```python
from build123d import *

# Parameters (mm, degrees)
CROQUIS1_R              = 2.159
CROQUIS1_W              = 21.082
CROQUIS1_H              = 21.082
SALIENTE_EXTRUIR1_DEPTH = 4.445
REDONDEO1_R             = 3.175
REDONDEO2_R             = 1.016
CHAFL_N1_SIZE           = 0.508


with BuildPart() as part:
    # Croquis1 → Saliente-Extruir1 (new body)
    with BuildSketch(Plane(origin=(0, 0, 0), x_dir=(1, 0, 0), z_dir=(0, 1, 0))):
        with BuildLine():
            Line((11.504506555, 42.935402979), (5.259202996, 19.62761279))
            ThreePointArc((5.259202996, 19.62761279), (-14.368409794, -14.368409794), (19.62761279, 5.259202996))
            Line((19.62761279, 5.259202996), (42.935402979, 11.504506555))
            ThreePointArc((42.935402979, 11.504506555), (31.430896424, 31.430896424), (11.504506555, 42.935402979))
        make_face()
        with Locations(Location((22.86, 9.652, 0), (0, 0, 270))):
            Circle(CROQUIS1_R, mode=Mode.SUBTRACT)
        Rectangle(CROQUIS1_W, CROQUIS1_H, mode=Mode.SUBTRACT)
    extrude(amount=SALIENTE_EXTRUIR1_DEPTH)

    # Redondeo1
    redondeo1_edges = [part.edges().sort_by_distance(p)[0] for p in [
        (42.935402979, 2.2225, -11.504506555),
        (19.62761279, 2.2225, -5.259202996),
        (5.259202996, 2.2225, -19.62761279),
        (11.504506555, 2.2225, -42.935402979),
    ]]
    fillet(redondeo1_edges, radius=REDONDEO1_R)

    # Redondeo2
    redondeo2_edges = [part.edges().sort_by_distance(p)[0] for p in [
        (10.541, 2.2225, 10.541),
        (10.541, 2.2225, -10.541),
        (-10.541, 2.2225, -10.541),
        (-10.541, 2.2225, 10.541),
    ]]
    fillet(redondeo2_edges, radius=REDONDEO2_R)

    # Chaflán1
    chafl_n1_edges = [part.edges().sort_by_distance(p)[0] for p in [
        (22.86, 0, -11.811),
        (22.86, 4.445, -11.811),
    ]]
    chamfer(chafl_n1_edges, length=CHAFL_N1_SIZE)


solid = part.part
```
Work out the finished part from the listing and answer in its coordinate system (mm). A direction names the side the tool comes from. Coordinates: 2 decimals unless noted, no trailing zeros. Loops run counter-clockwise (first coordinate to the right, second up) from the corner with the lowest first, then second, coordinate; pieces in that order, holes last.
1) Section D-D (z = -18.5) is taken. Give the vertices of the cut face in (x, y) (1 decimal), plus the area to 3 significant figures.
Results:
outline: (-8.4, 0) - (40.4, 0) - (40.4, 4.4) - (-8.4, 4.4) - close
area: 217 mm2
2) For faces 1 (the cylindrical face through (41.754, 2.254, -12.27)), 2 (the flat face through (10.541, 2, 0)), determine the directions among +Z, -Z, +X, -X, +Y, -Y from which every point of the face is accessible in a straight line to the end or side of a thin tool.
Results:
face 1: +X, +Y, -Y
face 2: +Y, -Y
3) Section A-A (z = 0) is taken. Give the vertices of the cut face in (x, y) (3 decimals), plus the area to 3 significant figures.
Results:
outline: (-20.32, 0) - (-10.541, 0) - (-10.541, 4.445) - (-20.32, 4.445) - close; (10.541, 0) - (20.32, 0) - (20.32, 4.445) - (10.541, 4.445) - close
area: 86.9 mm2
4) Consider probe 1 along X at (y, z) = (1.45, 8); probe 2 along X at (y, z) = (3.9, 8.5); probe 3 along Z at (x, y) = (4.5, 3.65). Determine where each line is inside the solid, lowest interval first.
Results:
probe 1: x = -18.68 to -10.54, 10.54 to 18.68
probe 2: x = -18.46 to -10.54, 10.54 to 18.46
probe 3: z = -20.53 to -10.54, 10.54 to 19.82
5) For a pull along X with two mould halves and no side action, classify faces 3 (the flat face through (-10.541, 2, 0)), 4 (the cylindrical face through (20.655, 2.254, -4.702)), 5 (the cylindrical face through (25, 2.2, -9.93)), 6 (the flat face through (8.37, 2.19, -31.24)) as +X half, -X half, draft (parallel to the pull), parting line (faces both ways), or undercut.
Results:
face 3: undercut
face 4: +X half
face 5: undercut
face 6: -X half
6) Flat-ended cylindrical pins translate along their axes: pin 1 (1 mm diameter, centred on x = -3.5, y = 3, fed in from +Z); pin 2 (1.3 mm diameter, centred on y = 2, z = -1.5, fed in from -X); pin 3 (2 mm diameter, centred on x = -4.5, y = 1.5, fed in from +Z); pin 4 (2.5 mm diameter, centred on x = 22.86, z = -9.652, fed in from +Y). Find the tip coordinate at first contact, or state that the pin passes through.
Results:
pin 1: stops at z = 20.1
pin 2: stops at x = -20.3
pin 3: stops at z = 20.02
pin 4: passes through
7) Section C-C (y = 1.9) is taken. Give the vertices of the cut face in (x, z) (3 decimals).
Results:
outline: (2.559, -20.158) arc R3.175 cw to (6.025, -22.486) - (10.651, -39.75) arc R3.175 ccw to (14.773, -41.923) arc R44.45 ccw to (41.923, -14.773) arc R3.175 ccw to (39.75, -10.651) - (22.486, -6.025) arc R3.175 cw to (20.158, -2.559) arc R20.32 ccw (long way) to start; hole (-10.541, -9.525) arc R1.016 ccw to (-9.525, -10.541) - (9.525, -10.541) arc R1.016 ccw to (10.541, -9.525) - (10.541, 9.525) arc R1.016 ccw to (9.525, 10.541) - (-9.525, 10.541) arc R1.016 ccw to (-10.541, 9.525) - close; hole circle Ø4.318 at (22.86, -9.652)
8) Section B-B (x = -7) is taken. Give the vertices of the cut face in (y, z) (3 decimals).
Results:
outline: (0, -19.076) - (4.445, -19.076) - (4.445, -10.541) - (0, -10.541) - close; (0, 10.541) - (4.445, 10.541) - (4.445, 19.076) - (0, 19.076) - close
